from build123d import *

# Parameters (mm, degrees)
SKETCH1_R           = 10
BOSS_EXTRUDE1_DEPTH = 10
CUT_EXTRUDE1_DEPTH  = 10
SKETCH3_W           = 14.282856858
SKETCH3_H           = 10
BOSS_EXTRUDE2_DEPTH = 150
SKETCH4_R           = 6.11
CUT_EXTRUDE2_DEPTH  = 10
FILLET1_R           = 5
FILLET2_R           = 2


with BuildPart() as part:
    # Sketch1 → Boss-Extrude1 (new body)
    with BuildSketch(Plane.XY):
        Circle(SKETCH1_R)
        with BuildLine():
            ThreePointArc((-1.666643333, 2.72), (0, -3.19), (1.666643333, 2.72))
            Line((1.666643333, 2.72), (-1.666643333, 2.72))
        make_face(mode=Mode.SUBTRACT)
    extrude(amount=BOSS_EXTRUDE1_DEPTH)

    # Sketch2 → Cut-Extrude1 (cut)
    with BuildSketch(Plane(origin=(0, 0, 0), x_dir=(-1, 0, 0), z_dir=(0, 0, -1))):
        with BuildLine():
            Line((7.141428429, -7), (-7.141428429, -7))
            ThreePointArc((-7.141428429, -7), (-3.872983346, -9.219544457), (0, -10))
            ThreePointArc((0, -10), (3.872983346, -9.219544457), (7.141428429, -7))
        make_face()
    extrude(amount=-CUT_EXTRUDE1_DEPTH, mode=Mode.SUBTRACT)

    # Sketch3 → Boss-Extrude2 (add)
    with BuildSketch(Plane.XZ.offset(7)):
        with Locations((0, 5)):
            Rectangle(SKETCH3_W, SKETCH3_H)
    extrude(amount=BOSS_EXTRUDE2_DEPTH)

    # Sketch4 → Cut-Extrude2 (cut)
    with BuildSketch(Plane(origin=(0, 0, 0), x_dir=(-1, 0, 0), z_dir=(0, 0, -1))):
        with Locations((0, -150)):
            Circle(SKETCH4_R)
    extrude(amount=-CUT_EXTRUDE2_DEPTH, mode=Mode.SUBTRACT)

    # Fillet1
    fillet1_edges = [part.edges().sort_by_distance(p)[0] for p in [
        (7.141428429, -7, 5),
        (-7.141428429, -7, 5),
    ]]
    fillet(fillet1_edges, radius=FILLET1_R)

    # Fillet2
    fillet2_edges = [part.edges().sort_by_distance(p)[0] for p in [
        (-7.141428429, -157, 5),
        (7.141428429, -157, 5),
    ]]
    fillet(fillet2_edges, radius=FILLET2_R)


solid = part.part
The model under review builds one solid part; all positions refer to its coordinate system, in mm. A direction names the side the tool comes from. Give positions to 0.01 mm unless a question says otherwise; leave off trailing zeros. Order: outer loops, then holes, each group sorted by start corner. A loop starts at its lowest first (then second) coordinate and runs counter-clockwise, first axis right, second up. Notation, with made-up numbers: M 78.5,-13.75 L 137.5,-13.75 A16 ccw 137.5,13.25 Z; hole C -30.5,-27.5 d2. An arc over 180 degrees is marked long. One line per question, with ' | ' between items. Start each with the question number.
1) Consider section A-A, the plane y = -150. Give the boundary of the cut face in (x, z), then the cut area to 3 significant figures.
2) Consider section D-D, the plane y = 0. Give the boundary of the cut face in (x, z).
3) Consider section C-C, the plane x = 0. Give the boundary of the cut face in (y, z).
4) Mouldability with a two-part tool opening along X and no side actions: class faces 4 (the face through (0, 10, 5)), 5 (the face through (-7.141, -81, 5)), 6 (the face through (1.325, -155.965, 4.93)) as pulls with the +X half, pulls with the -X half, needs draft (parallel to the pull), parting line crosses it, or undercut.
5) Consider section B-B, the plane z = 6.5. Give the boundary of the cut face in (x, y).
6) For faces 1 (the face through (7.141, -81, 5)), 2 (the face through (0, -72, 10)), 3 (the face through (0, 2.72, 5)), list the 3-axis set-ups (+Z, -Z, +X, -X, +Y, -Y) from which the entire face can be reached by the end or side of a thin tool; tool diameter is ignored.
7) Clearance check with flat-ended pins moving along their axes: P1, Ø3, axis at x = -6, z = 3.5, coming from the +Y side; P2, Ø5, axis at y = -78.5, z = 4.5, coming from the -X side; P3, Ø1, axis at x = -6.5, z = 6, coming from the -Y side. State where each tip first meets the part, or that it passes through.
8) Wall thickness on L1, parallel to Y at x = 0, z = 2.5; L2, parallel to X at y = 0, z = 2.25; L3, parallel to X at y = -89, z = 6.25: over which ranges is each line inside the solid? List them lowest first. Write a range as from..to.
Found:
1) outline: M -7.14,0 L -6.11,0 L -6.11,10 L -7.14,10 Z; M 6.11,0 L 7.14,0 L 7.14,10 L 6.11,10 Z | area: 20.6 mm²
2) outline: M -10,0 L -3.19,0 L -3.19,10 L -10,10 Z; M 3.19,0 L 10,0 L 10,10 L 3.19,10 Z
3) outline: M -157,0 L -156.11,0 L -156.11,10 L -157,10 Z; M -143.89,0 L -3.19,0 L -3.19,10 L -143.89,10 Z; M 2.72,0 L 10,0 L 10,10 L 2.72,10 Z
4) face 4: parting line crosses it | face 5: pulls with the -X half | face 6: undercut
5) outline: M -8.09,-5.87 A5 cw -7.14,-8.81 L -7.14,-155 A2 ccw -5.14,-157 L 5.14,-157 A2 ccw 7.14,-155 L 7.14,-8.81 A5 cw 8.09,-5.87 A10 ccw long Z; hole C 0,-150 d12.22; hole M -1.67,2.72 A3.19 ccw long 1.67,2.72 Z
6) face 1: +Z, -Z, +X, -Y | face 2: +Z, +X, -X, +Y, -Y | face 3: +Z, -Z
7) P1: stops at y = 8.93 | P2: stops at x = -7.14 | P3: stops at y = -156.81
8) L1: y = -157..-156.11, -143.89..-3.19, 2.72..10 | L2: x = -10..-3.19, 3.19..10 | L3: x = -7.14..7.14
